The listing builds one solid part. Answer for the finished solid, in the listing's coordinates (mm). Face numbers are marked on the shaded views. A direction names the side the tool comes from. Coordinates: 2 decimals unless noted, no trailing zeros. Loops run counter-clockwise (first coordinate to the right, second up) from the corner with the lowest first, then second, coordinate; pieces in that order, holes last. Notation, with made-up numbers: (11, 26) - (49, 26) arc R21 ccw to (49, 36) - close; hole circle Ø6 at (9, -19). An arc over 180 degrees is marked (long way). Put each result on its own line as item: value.
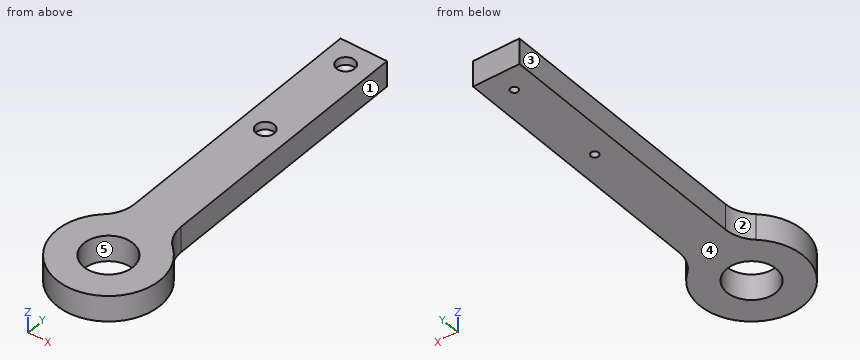
```python
from build123d import *

# Parameters (mm, degrees)
CYLINDER003_R     = 3.5
CYLINDER003_DEPTH = 10
CYLINDER002_R     = 1.5
CYLINDER002_DEPTH = 10
CYLINDER_R        = 9.5
CYLINDER_DEPTH    = 10
CYLINDER001_R     = 20
CYLINDER001_DEPTH = 10
BOX_W             = 18
BOX_H             = 110
BOX_DEPTH         = 10
FILLET_R          = 13


with BuildPart() as cylinder003:
    # Cylinder003 → Cylinder003 (new body)
    with BuildSketch(Plane(origin=(15, -5, 8), x_dir=(1, 0, 0), z_dir=(0, 0, 1))):
        Circle(CYLINDER003_R)
    extrude(amount=CYLINDER003_DEPTH)


with BuildPart() as cone:
    # Cone → Cone (revolve)
    with BuildSketch(Plane(origin=(15, -5, 6), x_dir=(1, 0, 0), z_dir=(0, -1, 0))):
        Polygon((0, 0), (1.5, 0), (3.5, 2), (0, 2), align=None)
    revolve(axis=Axis((15, -5, 6), (0, 0, 1)))


with BuildPart() as cylinder002:
    # Cylinder002 → Cylinder002 (new body)
    with BuildSketch(Plane(origin=(15, -5, 0), x_dir=(1, 0, 0), z_dir=(0, 0, 1))):
        Circle(CYLINDER002_R)
    extrude(amount=CYLINDER002_DEPTH)


with BuildPart() as fusion001:
    # Fusion001 base: copy of Cylinder002
    add(cylinder002.part)

    # Fusion001: union Cylinder003, Cone
    add(cylinder003.part)
    add(cone.part)


with BuildPart() as fusion001_1:
    # Fusion001 placement: moved
    add(fusion001.part.moved(Location((-15, 123, -1))))


with BuildPart() as fusion002:
    # Fusion002 base: copy of Cylinder002
    add(cylinder002.part)

    # Fusion002: union Cylinder003, Cone
    add(cylinder003.part)
    add(cone.part)


with BuildPart() as fusion002_1:
    # Fusion002 placement: moved
    add(fusion002.part.moved(Location((-15, 83, -1))))


with BuildPart() as fusion003:
    # Cylinder → Cylinder (new body)
    with BuildSketch(Plane.XY):
        Circle(CYLINDER_R)
    extrude(amount=CYLINDER_DEPTH)

    # Fusion003: union Fusion001, Fusion002
    add(fusion001_1.part)
    add(fusion002_1.part)


with BuildPart() as cylinder001:
    # Cylinder001 → Cylinder001 (new body)
    with BuildSketch(Plane.XY):
        Circle(CYLINDER001_R)
    extrude(amount=CYLINDER001_DEPTH)


with BuildPart() as cut:
    # Box → Box (new body)
    with BuildSketch(Plane(origin=(-9, 17, 0), x_dir=(1, 0, 0), z_dir=(0, 0, 1))):
        with Locations((9, 55)):
            Rectangle(BOX_W, BOX_H)
    extrude(amount=BOX_DEPTH)

    # Fusion: union Cylinder001
    add(cylinder001.part)

    # Fillet
    fillet_edges = [cut.edges().sort_by_distance(p)[0] for p in [
        (9, 17.860571, 5),
        (-9, 17.860571, 5),
    ]]
    fillet(fillet_edges, radius=FILLET_R)

    # Cut: cut Fusion003
    add(fusion003.part, mode=Mode.SUBTRACT)


solid = cut.part
```
1) The part is cut by section C-C (x = -7). Give the vertices of the cut face in (y, z) (3 decimals).
Found:
outline: (-18.735, 0) - (-6.423, 0) - (-6.423, 10) - (-18.735, 10) - close; (6.423, 0) - (127, 0) - (127, 10) - (6.423, 10) - close
2) The part is cut by section D-D (y = -6). Give the vertices of the cut face in (x, z), and give its area (3 significant figures).
Found:
outline: (-19.08, 0) - (-7.37, 0) - (-7.37, 10) - (-19.08, 10) - close; (7.37, 0) - (19.08, 0) - (19.08, 10) - (7.37, 10) - close
area: 234 mm^2
3) Straight lines are drawn through the part: L1, parallel to Y at x = 0, z = 1.65; L2, parallel to Y at x = 0, z = 8.2; L3, parallel to X at y = 78, z = 8.25. For each, find the intervals that lie inside material, in ascending order. Write a range as [from, to].
Found:
L1: y = [-20, -9.5], [9.5, 76.5], [79.5, 116.5], [119.5, 127]
L2: y = [-20, -9.5], [9.5, 74.5], [81.5, 114.5], [121.5, 127]
L3: x = [-9, -3.5], [3.5, 9]
4) Each of these flat-tipped pins is pushed along its axis until it touches: pin 1 (1 mm diameter, centred on x = 10.5, z = 4, fed in from -Y); pin 2 (5 mm diameter, centred on y = 37.5, z = 6.5, fed in from +X); pin 3 (6 mm diameter, centred on y = 112, z = 5, fed in from -X); pin 4 (15 mm diameter, centred on x = 0, y = 0, fed in from +Z). Where does it stop, or does it pass through?
Found:
pin 1: stops at y = -17.32
pin 2: stops at x = 9
pin 3: stops at x = -9
pin 4: passes through
5) For the marked faces 1 and 2, determine the directions among +Z, -Z, +X, -X, +Y, -Y from which every point of the face is accessible in a straight line to the end or side of a thin tool.
Found:
face 1: +Z, -Z, +X, +Y
face 2: +Z, -Z, -X, +Y
6) The part is cut by section A-A (y = 78). Give the vertices of the cut face in (x, z), and give its area (3 significant figures).
Found:
outline: (-9, 0) - (-1.5, 0) - (-1.5, 5) - (-3.5, 7) - (-3.5, 10) - (-9, 10) - close; (1.5, 0) - (9, 0) - (9, 10) - (3.5, 10) - (3.5, 7) - (1.5, 5) - close
area: 134 mm^2
7) The part is cut by section B-B (x = 0). Give the vertices of the cut face in (y, z), and give its area (3 significant figures).
Found:
outline: (-20, 0) - (-9.5, 0) - (-9.5, 10) - (-20, 10) - close; (9.5, 0) - (76.5, 0) - (76.5, 5) - (74.5, 7) - (74.5, 10) - (9.5, 10) - close; (79.5, 0) - (116.5, 0) - (116.5, 5) - (114.5, 7) - (114.5, 10) - (81.5, 10) - (81.5, 7) - (79.5, 5) - close; (119.5, 0) - (127, 0) - (127, 10) - (121.5, 10) - (121.5, 7) - (119.5, 5) - close
area: 1,190 mm^2
8) For a pull along X with two mould halves and no side action, classify the marked faces 3, 4 and 5 as pulls with the +X half, pulls with the -X half, needs draft (parallel to the pull), parting line crosses it, or undercut.
Found:
face 3: pulls with the -X half
face 4: needs draft
face 5: undercut
